```python
from build123d import *

# Parameters (mm, degrees)
SKETCH1_W               = 110
SKETCH1_H               = 54
BOSS_EXTRUDE1_DEPTH     = 3
SKETCH2_W               = 34
SKETCH2_H               = 28.5
BOSS_EXTRUDE2_DEPTH     = 50.5
CUT_EXTRUDE1_DEPTH      = 125.013104146
CUT_EXTRUDE1_DEPTH_BACK = 125.013104146
SKETCH3_R               = 10.25
CUT_EXTRUDE2_DEPTH      = 86.304234948
CUT_EXTRUDE2_DEPTH_BACK = 86.304234948
SKETCH4_W               = 22
SKETCH4_H               = 30
FILLET1_R               = 10
SKETCH5_W               = 34
SKETCH5_H               = 28.5
BOSS_EXTRUDE3_DEPTH     = 44
CUT_EXTRUDE3_DEPTH      = 92.995923823
CUT_EXTRUDE3_DEPTH_BACK = 92.995923823
SKETCH6_R               = 10.25


with BuildPart() as part:
    # Sketch1 → Boss-Extrude1 (new body)
    with BuildSketch(Plane(origin=(0, 0, 0), x_dir=(1, 0, 0), z_dir=(0, 1, 0))):
        Rectangle(SKETCH1_W, SKETCH1_H)
    extrude(amount=BOSS_EXTRUDE1_DEPTH)

    # Sketch2 → Boss-Extrude2 (add)
    with BuildSketch(Plane.XZ):
        with Locations((38, 0)):
            Rectangle(SKETCH2_W, SKETCH2_H)
        with Locations((-38, 0)):
            Rectangle(SKETCH2_W, SKETCH2_H)
    extrude(amount=BOSS_EXTRUDE2_DEPTH)

    # Sketch3 → Cut-Extrude1 (cut, two sides: drawn at the far end of the back side and taken through both)
    with BuildSketch(Plane(origin=(55, 0, 0), x_dir=(0, 0, -1), z_dir=(1, 0, 0)).offset(-CUT_EXTRUDE1_DEPTH_BACK)):
        with Locations((0, -39.25)):
            Circle(SKETCH3_R)
    extrude(amount=CUT_EXTRUDE1_DEPTH + CUT_EXTRUDE1_DEPTH_BACK, mode=Mode.SUBTRACT)

    # Sketch4 → Cut-Extrude2 (cut, two sides: drawn at the far end of the back side and taken through both)
    with BuildSketch(Plane.XY.offset(14.25).offset(-CUT_EXTRUDE2_DEPTH_BACK)):
        with Locations((38, -35.5)):
            Rectangle(SKETCH4_W, SKETCH4_H)
        with Locations((-38, -35.5)):
            Rectangle(SKETCH4_W, SKETCH4_H)
    extrude(amount=CUT_EXTRUDE2_DEPTH + CUT_EXTRUDE2_DEPTH_BACK, mode=Mode.SUBTRACT)

    # Fillet1
    fillet1_edges = [part.edges().sort_by_distance(p)[0] for p in [
        (52, -50.5, 14.25),
        (24, -50.5, -14.25),
        (-24, -50.5, 14.25),
        (-52, -50.5, -14.25),
        (-52, -50.5, 14.25),
        (-24, -50.5, -14.25),
        (24, -50.5, 14.25),
        (52, -50.5, -14.25),
    ]]
    fillet(fillet1_edges, radius=FILLET1_R)

    # Sketch5 → Boss-Extrude3 (add)
    with BuildSketch(Plane(origin=(0, 3, 0), x_dir=(1, 0, 0), z_dir=(0, 1, 0))):
        Rectangle(SKETCH5_W, SKETCH5_H)
    extrude(amount=BOSS_EXTRUDE3_DEPTH)

    # Sketch6 → Cut-Extrude3 (cut, two sides: drawn at the far end of the back side and taken through both)
    with BuildSketch(Plane(origin=(17, 0, 0), x_dir=(0, 0, -1), z_dir=(1, 0, 0)).offset(-CUT_EXTRUDE3_DEPTH_BACK)):
        with Locations((0, 35.75)):
            Circle(SKETCH6_R)
    extrude(amount=CUT_EXTRUDE3_DEPTH + CUT_EXTRUDE3_DEPTH_BACK, mode=Mode.SUBTRACT)


solid = part.part
```
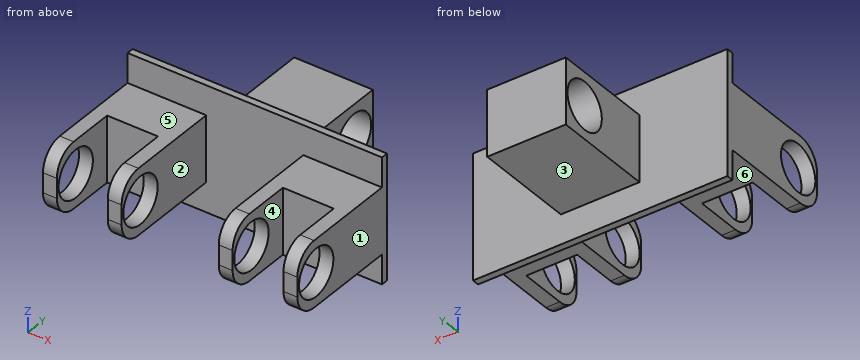
Part model, mm, in its own coordinate system. Face numbers are marked on the shaded views. A direction names the side the tool comes from. Round coordinates to 2 decimals unless told otherwise and drop trailing zeros. Write each loop counter-clockwise with the first axis right and the second up, starting at its lowest first coordinate (ties: lowest second). Pieces come first, ordered by that corner, then holes. Notation, with made-up numbers: M 19,27.5 L 69,27.5 A36 ccw 69,66.5 Z; hole C 12.25,32 d7. An arc over 180 degrees is marked long. One line per question, with ' | ' between items.
(1) Saw through at B-B on z = 0. Count the separate pieces of the cut face and the enclosed holes in it, then the cut area to 3 significant figures.
Answer key:
separate pieces: 6 | enclosed holes: 0 | area: 2,750 mm^2
(2) Two-plate mould, pull along X, no slides. Class the marked faces 1, 2 and 3: released by +X, released by -X, zero draft, split by the parting line, or undercut.
Answer key:
face 1: released by +X | face 2: undercut | face 3: zero draft
(3) Probe line 1 along X through (y, z) = (-18, -0.5); line 2 along Y through (x, z) = (51, 0); line 3 along Z through (x, y) = (-51.8, -39.25). List the from-to ranges inside material, lowest first.
Answer key:
line 1: x = -55 to -21, 21 to 55 | line 2: y = -50.5 to -49.5, -29 to 3 | line 3: z = -14.25 to -10.25, 10.25 to 14.25
(4) Saw through at C-C on x = 45. Write the cut outline in (y, z), then the cut area to 3 significant figures.
Answer key:
outline: M -20.5,-14.25 L 0,-14.25 L 0,-27 L 3,-27 L 3,27 L 0,27 L 0,14.25 L -20.5,14.25 Z | area: 746 mm^2
(5) Saw through at A-A on y = 35.75. Write the cut outline in (x, z).
Answer key:
outline: M -17,-14.25 L 17,-14.25 L 17,-10.25 L -17,-10.25 Z; M -17,10.25 L 17,10.25 L 17,14.25 L -17,14.25 Z
(6) 3-axis set-ups, long thin cutter, end or side, ignore diameter. For the marked faces 4, 5 and 6: which of +Z, -Z, +X, -X, +Y, -Y reach the whole face in a straight line?
Answer key:
face 4: +Z, -Z, -Y | face 5: +Z, +X, -X, -Y | face 6: -Z, +X, -X, -Y
(7) Saw through at D-D on y = -16.5. Write the cut outline in (x, z).
Answer key:
outline: M -55,-14.25 L -21,-14.25 L -21,14.25 L -55,14.25 Z; M 21,-14.25 L 55,-14.25 L 55,14.25 L 21,14.25 Z
(8) Pin check, flat tips, straight feed: pin 1 (6.5 mm diameter, centred on x = -43, z = -2, fed in from -Y); pin 2 (16 mm diameter, centred on x = 22, z = -3.5, fed in from +Y); pin 3 (5 mm diameter, centred on y = -17, z = 18.5, fed in from -X); pin 4 (10 mm diameter, centred on x = 34.5, y = -11.5, fed in from -Z). Stop position of each tip, or through.
Answer key:
pin 1: stops at y = -20.5 | pin 2: stops at y = 47 | pin 3: passes through | pin 4: stops at z = -14.25
